from build123d import *

# Parameters (mm, degrees)
SKETCH1_W           = 44
SKETCH1_H           = 14
SKETCH1_W_2         = 51
SKETCH1_H_2         = 2
SKETCH3_W           = 45
SKETCH3_H           = 2
SKETCH4_R           = 15
BOSS_EXTRUDE1_DEPTH = 6
SKETCH5_R           = 9.2
CUT_EXTRUDE3_DEPTH  = 7
SKETCH6_R           = 7
CUT_EXTRUDE4_DEPTH  = 27
FILLET1_R           = 2
SKETCH9_R           = 44
SKETCH9_R_2         = 38
CUT_EXTRUDE6_DEPTH  = 2
SKETCH13_R          = 38
SKETCH13_R_2        = 7
BOSS_EXTRUDE2_DEPTH = 6
FILLET5_R           = 1
SKETCH14_R          = 14
SKETCH14_R_2        = 7
CUT_EXTRUDE9_DEPTH  = 16
BOSS_EXTRUDE3_DEPTH = 9
SKETCH16_W          = 15
SKETCH16_H          = 10
SKETCH17_R          = 5
CUT_EXTRUDE11_DEPTH = 10
FILLET6_R           = 1
SKETCH26_W          = 3
SKETCH26_H          = 2
SKETCH29_R          = 48
SKETCH29_R_2        = 45
CUT_EXTRUDE12_DEPTH = 2
FILLET7_R           = 3
SKETCH34_R          = 5
SKETCH34_R_2        = 48
BOSS_EXTRUDE7_DEPTH = 8
CUT_EXTRUDE14_DEPTH = 8
CUT_EXTRUDE15_DEPTH = 18
SKETCH40_R          = 5
CUT_EXTRUDE16_DEPTH = 20
CUT_EXTRUDE17_DEPTH = 8


with BuildPart() as part:
    # Sketch1 → Revolve1 (revolve)
    with BuildSketch(Plane(origin=(0, 0, 0), x_dir=(0, 0, -1), z_dir=(1, 0, 0)), mode=Mode.PRIVATE) as revolve1_sk:
        with Locations((22, 25)):
            Rectangle(SKETCH1_W, SKETCH1_H)
        Polygon((44, 18), (0, 18), (0, 2), (51, 2), align=None)
        with Locations((25.5, 1)):
            Rectangle(SKETCH1_W_2, SKETCH1_H_2)
    revolve(revolve1_sk.sketch.rotate(Axis((0, 32.712152445, 0), (0, -1, 0)), 180), axis=Axis((0, 32.712152445, 0), (0, -1, 0)))

    # Sketch3 → Cut-Revolve1 (revolve, cut)
    with BuildSketch(Plane(origin=(0, 0, 0), x_dir=(0, 0, -1), z_dir=(1, 0, 0))):
        with Locations((22.5, 1)):
            Rectangle(SKETCH3_W, SKETCH3_H)
        Polygon((0, 18), (0, 2), (45, 2), (41, 18), align=None)
    revolve(axis=Axis((0, -18.749054984, 0), (0, 1, 0)), mode=Mode.SUBTRACT)

    # Sketch4 → Boss-Extrude1 (add)
    with BuildSketch(Plane(origin=(0, 18, 0), x_dir=(-1, 0, 0), z_dir=(0, -1, 0))):
        with Locations(Location((0, 0, 0), (0, 0, 90))):
            Circle(SKETCH4_R)
    extrude(amount=BOSS_EXTRUDE1_DEPTH)

    # Sketch5 → Cut-Extrude3 (cut)
    with BuildSketch(Plane.XZ.offset(-12)):
        with Locations(Location((0, 0, 0), (0, 0, 270))):
            Circle(SKETCH5_R)
    extrude(amount=-CUT_EXTRUDE3_DEPTH, mode=Mode.SUBTRACT)

    # Sketch6 → Cut-Extrude4 (cut)
    with BuildSketch(Plane.XZ.offset(-19)):
        with Locations(Location((0, 0, 0), (0, 0, 270))):
            Circle(SKETCH6_R)
    extrude(amount=-CUT_EXTRUDE4_DEPTH, mode=Mode.SUBTRACT)

    # Fillet1
    fillet1_edges = [part.edges().sort_by_distance(p)[0] for p in [
        (0, 19, 9.2),
    ]]
    fillet(fillet1_edges, radius=FILLET1_R)

    # Sketch9 → Cut-Extrude6 (cut)
    with BuildSketch(Plane(origin=(0, 32, 0), x_dir=(1, 0, 0), z_dir=(0, 1, 0))):
        with Locations(Location((0, 0, 0), (0, 0, 270))):
            Circle(SKETCH9_R)
        with Locations(Location((0, 0, 0), (0, 0, 270))):
            Circle(SKETCH9_R_2, mode=Mode.SUBTRACT)
    extrude(amount=-CUT_EXTRUDE6_DEPTH, mode=Mode.SUBTRACT)

    # Sketch13 → Boss-Extrude2 (add)
    with BuildSketch(Plane(origin=(0, 32, 0), x_dir=(1, 0, 0), z_dir=(0, 1, 0))):
        with Locations(Location((0, 0, 0), (0, 0, 270))):
            Circle(SKETCH13_R)
        with Locations(Location((0, 0, 0), (0, 0, 90))):
            Circle(SKETCH13_R_2, mode=Mode.SUBTRACT)
    extrude(amount=BOSS_EXTRUDE2_DEPTH)

    # Fillet5
    fillet5_edges = [part.edges().sort_by_distance(p)[0] for p in [
        (0, 38, -38),
    ]]
    fillet(fillet5_edges, radius=FILLET5_R)

    # Sketch14 → Cut-Extrude9 (cut)
    with BuildSketch(Plane(origin=(0, 38, 0), x_dir=(1, 0, 0), z_dir=(0, 1, 0))):
        with Locations(Location((0, 0, 0), (0, 0, 270))):
            Circle(SKETCH14_R)
        with Locations(Location((0, 0, 0), (0, 0, 90))):
            Circle(SKETCH14_R_2, mode=Mode.SUBTRACT)
    extrude(amount=-CUT_EXTRUDE9_DEPTH, mode=Mode.SUBTRACT)

    # Sketch15 → Boss-Extrude3 (add)
    with BuildSketch(Plane(origin=(0, 0, 0), x_dir=(1, 0, 0), z_dir=(0, 1, 0))):
        with BuildLine():
            Line((-77.642135624, -34.142135624), (-34.142135624, -77.642135624))
            ThreePointArc((-34.142135624, -77.642135624), (-27.653668647, -81.97759065), (-20, -83.5))
            Line((-20, -83.5), (20, -83.5))
            ThreePointArc((20, -83.5), (27.653668647, -81.97759065), (34.142135624, -77.642135624))
            Line((34.142135624, -77.642135624), (55.785028834, -51.421252812))
            ThreePointArc((55.785028834, -51.421252812), (74.5, 0), (55.785028834, 51.421252812))
            Line((55.785028834, 51.421252812), (36.56649078, 74.704971363))
            ThreePointArc((36.56649078, 74.704971363), (29.3781814, 81.164928917), (20, 83.5))
            Line((20, 83.5), (-20, 83.5))
            ThreePointArc((-20, 83.5), (-27.653668647, 81.97759065), (-34.142135624, 77.642135624))
            Line((-34.142135624, 77.642135624), (-77.642135624, 34.142135624))
            ThreePointArc((-77.642135624, 34.142135624), (-81.97759065, 27.653668647), (-83.5, 20))
            Line((-83.5, 20), (-83.5, -20))
            ThreePointArc((-83.5, -20), (-81.97759065, -27.653668647), (-77.642135624, -34.142135624))
        make_face()
    extrude(amount=BOSS_EXTRUDE3_DEPTH)

    # Sketch16 → Cut-Revolve3 (revolve, cut)
    with BuildSketch(Plane(origin=(0, 0, 0), x_dir=(0, 0, -1), z_dir=(1, 0, 0))):
        Polygon((15, 12), (15, 2), (48, 2), (41, 18), (15, 18), align=None)
        with Locations((7.5, 7)):
            Rectangle(SKETCH16_W, SKETCH16_H)
        Polygon((0, 2), (0, 0), (48, 0), (48, 2), (15, 2), align=None)
    revolve(axis=Axis((0, -11.590018377, 0), (0, 1, 0)), mode=Mode.SUBTRACT)

    # Sketch17 → Cut-Extrude11 (cut)
    with BuildSketch(Plane(origin=(0, 0, 0), x_dir=(-1, 0, 0), z_dir=(0, -1, 0))):
        with Locations(Location((0, 70, 0), (0, 0, 90))):
            Circle(SKETCH17_R)
        with Locations(Location((0, -70, 0), (0, 0, 90))):
            Circle(SKETCH17_R)
    extrude(amount=-CUT_EXTRUDE11_DEPTH, mode=Mode.SUBTRACT)

    # Sketch21 → Revolve3 (revolve)
    with BuildSketch(Plane(origin=(0, 0, 0), x_dir=(0, 0, -1), z_dir=(1, 0, 0)), mode=Mode.PRIVATE) as revolve3_sk:
        Polygon((40.904222375, 30), (45.904222375, 9), (49, 9), (44, 30), align=None)
    revolve(revolve3_sk.sketch.rotate(Axis((0, -11.272163733, 0), (0, 1, 0)), 180), axis=Axis((0, -11.272163733, 0), (0, 1, 0)))

    # Fillet6
    fillet6_edges = [part.edges().sort_by_distance(p)[0] for p in [
        (0, 30, -44),
    ]]
    fillet(fillet6_edges, radius=FILLET6_R)

    # Sketch26 → Revolve4 (revolve)
    with BuildSketch(Plane(origin=(0, 0, 0), x_dir=(0, 0, -1), z_dir=(1, 0, 0))):
        Polygon((48, 2), (45, 2), (41, 18), align=None)
        with Locations((46.5, 1)):
            Rectangle(SKETCH26_W, SKETCH26_H)
    revolve(axis=Axis((0, -14.846098764, 0), (0, 1, 0)))

    # Sketch29 → Cut-Extrude12 (cut)
    with BuildSketch(Plane(origin=(0, 0, 0), x_dir=(-1, 0, 0), z_dir=(0, -1, 0))):
        with Locations(Location((0, 0, 0), (0, 0, 90))):
            Circle(SKETCH29_R)
        Circle(SKETCH29_R_2, mode=Mode.SUBTRACT)
    extrude(amount=-CUT_EXTRUDE12_DEPTH, mode=Mode.SUBTRACT)

    # Fillet7
    fillet7_edges = [part.edges().sort_by_distance(p)[0] for p in [
        (0, 2, 45),
    ]]
    fillet(fillet7_edges, radius=FILLET7_R)

    # Sketch34 → Boss-Extrude7 (add)
    with BuildSketch(Plane.XZ):
        with BuildLine():
            Line((-77.642135624, -34.142135624), (-34.142135624, -77.642135624))
            ThreePointArc((-34.142135624, -77.642135624), (-27.653668647, -81.97759065), (-20, -83.5))
            Line((-20, -83.5), (20, -83.5))
            ThreePointArc((20, -83.5), (27.653668647, -81.97759065), (34.142135624, -77.642135624))
            Line((34.142135624, -77.642135624), (36.56649078, -74.704971363))
            Line((36.56649078, -74.704971363), (55.785028834, -51.421252812))
            ThreePointArc((55.785028834, -51.421252812), (74.5, 0), (55.785028834, 51.421252812))
            Line((55.785028834, 51.421252812), (36.56649078, 74.704971362))
            Line((36.56649078, 74.704971362), (34.142135624, 77.642135624))
            ThreePointArc((34.142135624, 77.642135624), (27.653668647, 81.97759065), (20, 83.5))
            Line((20, 83.5), (-20, 83.5))
            ThreePointArc((-20, 83.5), (-27.653668647, 81.97759065), (-34.142135624, 77.642135624))
            Line((-34.142135624, 77.642135624), (-77.642135624, 34.142135624))
            ThreePointArc((-77.642135624, 34.142135624), (-81.97759065, 27.653668647), (-83.5, 20))
            Line((-83.5, 20), (-83.5, -20))
            ThreePointArc((-83.5, -20), (-81.97759065, -27.653668647), (-77.642135624, -34.142135624))
        make_face()
        with Locations(Location((0, -70, 0), (0, 0, 270))):
            Circle(SKETCH34_R, mode=Mode.SUBTRACT)
        with Locations(Location((0, 0, 0), (0, 0, 270))):
            Circle(SKETCH34_R_2, mode=Mode.SUBTRACT)
        with Locations(Location((0, 70, 0), (0, 0, 270))):
            Circle(SKETCH34_R, mode=Mode.SUBTRACT)
    extrude(amount=BOSS_EXTRUDE7_DEPTH)

    # Sketch35 → Cut-Extrude14 (cut)
    with BuildSketch(Plane(origin=(0, -8, 0), x_dir=(-1, 0, 0), z_dir=(0, -1, 0))):
        Polygon((-9.814954576, 70), (-4.907477288, 61.5), (4.907477288, 61.5), (9.814954576, 70), (4.907477288, 78.5), (-4.907477288, 78.5), align=None)
        Polygon((-9.814954576, -70), (-4.907477288, -78.5), (4.907477288, -78.5), (9.814954576, -70), (4.907477288, -61.5), (-4.907477288, -61.5), align=None)
    extrude(amount=-CUT_EXTRUDE14_DEPTH, mode=Mode.SUBTRACT)

    # Sketch36 → Cut-Extrude15 (cut)
    with BuildSketch(Plane(origin=(0, 38, 0), x_dir=(1, 0, 0), z_dir=(0, 1, 0))):
        with BuildLine():
            ThreePointArc((28.5, 0), (26, 2.5), (23.5, 0))
            Line((23.5, 0), (28.5, 0))
        make_face()
        with BuildLine():
            Line((28.5, 0), (23.5, 0))
            ThreePointArc((23.5, 0), (26, -2.5), (28.5, 0))
        make_face()
        with BuildLine():
            ThreePointArc((-28.5, 0), (-26, -2.5), (-23.5, 0))
            Line((-23.5, 0), (-28.5, 0))
        make_face()
        with BuildLine():
            Line((-28.5, 0), (-23.5, 0))
            ThreePointArc((-23.5, 0), (-26, 2.5), (-28.5, 0))
        make_face()
    extrude(amount=-CUT_EXTRUDE15_DEPTH, mode=Mode.SUBTRACT)

    # Sketch40 → Cut-Extrude16 (cut)
    with BuildSketch(Plane.XZ.offset(8)):
        with Locations(Location((-70, 0, 0), (0, 0, 270))):
            Circle(SKETCH40_R)
    extrude(amount=-CUT_EXTRUDE16_DEPTH, mode=Mode.SUBTRACT)

    # Sketch41 → Cut-Extrude17 (cut)
    with BuildSketch(Plane(origin=(0, -8, 0), x_dir=(-1, 0, 0), z_dir=(0, -1, 0))):
        Polygon((70, 9.814954576), (61.5, 4.907477288), (61.5, -4.907477288), (70, -9.814954576), (78.5, -4.907477288), (78.5, 4.907477288), align=None)
    extrude(amount=-CUT_EXTRUDE17_DEPTH, mode=Mode.SUBTRACT)


solid = part.part
Verification items for the finished model (mm, model axes). A direction names the side the tool comes from. Coordinates: 2 decimals unless noted, no trailing zeros. Order: outer loops, then holes, each group sorted by start corner. A loop starts at its lowest first (then second) coordinate and runs counter-clockwise, first axis right, second up. Notation, with made-up numbers: M 66,-12 L 115,-12 A35 ccw 115,20 Z; hole C -13.75,88 d1. An arc over 180 degrees is marked long. One line per item, written item: value. Start each with the question number.
Item 1: Sectioned sample at C-C on z = 72.5. Record the cut outline in (x, y).
Item 2: Thickness scan on probe 1 along Z at (x, y) = (4.5, 5.5); probe 2 along Y at (x, z) = (44, -43.5); probe 3 along Y at (x, z) = (-35, 1). Record the ranges inside material, lowest first.
Item 3: Mould release check, pull along Z, two halves, no side actions. Record for faces 1 (the flat face through (-1, 18, -18)), 2 (the flat face through (-41, 9, 36)), 3 (the cylindrical face through (-27.755, 0.619, -81.935)): pulls with the +Z half, pulls with the -Z half, needs draft (parallel to the pull), parting line crosses it, or undercut.
Item 4: Access from +Z, -Z, +X, -X, +Y, -Y to the whole of each face (thin tool, end or side, straight path). Record for faces 4 (the flat face through (-74.19, -4.056, 7.396)), 5 (the cylindrical face through (-1.915, 4.437, -74.619)).
Item 5: Sectioned sample at B-B on y = 33. Record the cut outline in (x, z).
Item 6: Depth check by flat-ended pin: P1, Ø6, axis at y = 17, z = 13.5, coming from the -X side; P2, Ø6, axis at x = -26, z = 0, coming from the +Y side; P3, Ø6, axis at y = 11, z = -53.5, coming from the +X side; P4, Ø14.5, axis at x = 0, z = 0, coming from the -Y side. Enter the tip coordinate at first touch or a pass-through.
Item 7: Sectioned sample at A-A on z = 0. Give the number of separate pieces and of enclosed holes in the cut face, then the cut area to 3 significant figures.
Calculated:
1. outline: M -39.28,-8 L -8.37,-8 L -8.37,0 L -4.33,0 L -4.33,9 L -39.28,9 Z; M 4.33,0 L 8.37,0 L 8.37,-8 L 38.39,-8 L 38.39,9 L 4.33,9 Z
2. probe 1: -83.5 to -72.18, -67.82 to -43.89, 43.89 to 67.82, 72.18 to 83.5
2. probe 2: -8 to 9
2. probe 3: 18 to 38
3. face 1: undercut
3. face 2: needs draft
3. face 3: pulls with the -Z half
4. face 4: -Y
4. face 5: +Y, -Y
5. outline: C 0,0 d76; hole C -26,0 d5; hole C 0,0 d28; hole C 26,0 d5
6. P1: x = -46.22
6. P2: y = 38
6. P3: x = 55.92
6. P4: y = 19
7. separate pieces: 3
7. enclosed holes: 0
7. area: 2,070 mm^2
